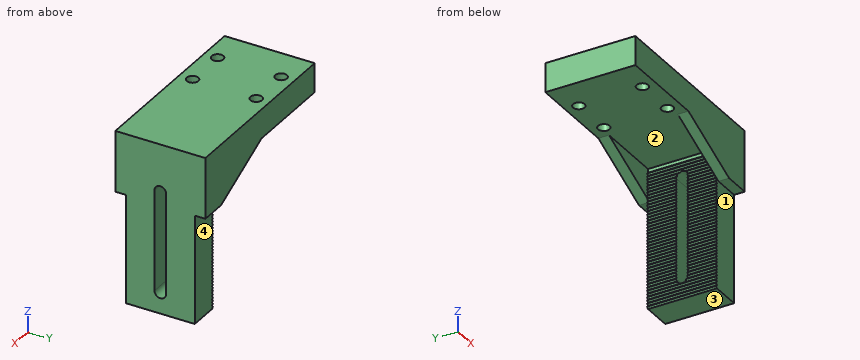
```python
from build123d import *

# Parameters (mm, degrees)
EXTRUDE_1_DEPTH          = 17
SKETCH_4_R               = 1.1
CUT_EXTRUDE_2_DEPTH      = 51.378566871
SKETCH_8_W               = 20.5
SKETCH_8_H               = 2
CUT_EXTRUDE_5_DEPTH      = 48.042533945
EXTRUDE_2_DEPTH          = 13
CUT_EXTRUDE_4_DEPTH      = 10
CUT_EXTRUDE_4_DEPTH_BACK = 48.042533945
EXTRUDE_3_DEPTH          = 2
EXTRUDE_4_DEPTH          = 2


with BuildPart() as part:
    # 草图1 → 凸台-拉伸1 (new body)
    with BuildSketch(Plane(origin=(0, 0, 0), x_dir=(1, 0, 0), z_dir=(0, 1, 0))):
        Polygon((0, 0), (-35, 0), (-35, 5.5), (-5, 5.5), (-5, 32), (0, 32), align=None)
    extrude(amount=EXTRUDE_1_DEPTH)

    # 草图4 → 切除-拉伸2 (cut, through all)
    with BuildSketch(Plane.XY):
        with Locations((-28.5, 14.5)):
            Circle(SKETCH_4_R)
        with Locations((-20.5, 14.5)):
            Circle(SKETCH_4_R)
        with Locations((-28.5, 2.5)):
            Circle(SKETCH_4_R)
        with Locations((-20.5, 2.5)):
            Circle(SKETCH_4_R)
    extrude(amount=-CUT_EXTRUDE_2_DEPTH, mode=Mode.SUBTRACT)

    # 草图8 → 切除-拉伸5 (cut, through all)
    with BuildSketch(Plane.ZY.offset(5)):
        with Locations((-21.75, 16)):
            Rectangle(SKETCH_8_W, SKETCH_8_H)
        with Locations((-21.75, 1)):
            Rectangle(SKETCH_8_W, SKETCH_8_H)
    extrude(amount=-CUT_EXTRUDE_5_DEPTH, mode=Mode.SUBTRACT)

    # 草图11 → 凸台-拉伸2 (add)
    with BuildSketch(Plane.XZ.offset(-2)):
        Polygon((-5, -5.5), (-5, -32), (-5.5, -32), (-5.8, -31.7), (-5.5, -31.4), (-5.8, -31.1), (-5.5, -30.8), (-5.8, -30.5), (-5.5, -30.2), (-5.8, -29.9), (-5.5, -29.6), (-5.8, -29.3), (-5.5, -29), (-5.8, -28.7), (-5.5, -28.4), (-5.8, -28.1), (-5.5, -27.8), (-5.8, -27.5), (-5.5, -27.2), (-5.8, -26.9), (-5.5, -26.6), (-5.8, -26.3), (-5.5, -26), (-5.8, -25.7), (-5.5, -25.4), (-5.8, -25.1), (-5.5, -24.8), (-5.8, -24.5), (-5.5, -24.2), (-5.8, -23.9), (-5.5, -23.6), (-5.8, -23.3), (-5.5, -23), (-5.8, -22.7), (-5.5, -22.4), (-5.8, -22.1), (-5.5, -21.8), (-5.8, -21.5), (-5.5, -21.2), (-5.8, -20.9), (-5.5, -20.6), (-5.8, -20.3), (-5.5, -20), (-5.8, -19.7), (-5.5, -19.4), (-5.8, -19.1), (-5.5, -18.8), (-5.8, -18.5), (-5.5, -18.2), (-5.8, -17.9), (-5.5, -17.6), (-5.8, -17.3), (-5.5, -17), (-5.8, -16.7), (-5.5, -16.4), (-5.8, -16.1), (-5.5, -15.8), (-5.8, -15.5), (-5.5, -15.2), (-5.8, -14.9), (-5.5, -14.6), (-5.8, -14.3), (-5.5, -14), (-5.8, -13.7), (-5.5, -13.4), (-5.8, -13.1), (-5.5, -12.8), (-5.8, -12.5), (-5.5, -12.2), (-5.8, -11.9), (-5.5, -11.6), (-5.8, -11.3), (-5.5, -11), (-5.8, -10.7), (-5.5, -10.4), (-5.8, -10.1), (-5.5, -9.8), (-5.8, -9.5), (-5.5, -9.2), (-5.8, -8.9), (-5.5, -8.6), (-5.8, -8.3), (-5.5, -8), (-5.8, -7.7), (-5.5, -7.4), (-5.8, -7.1), (-5.5, -6.8), (-5.8, -6.5), (-5.5, -6.2), (-5.5, -5.5), align=None)
    extrude(amount=-EXTRUDE_2_DEPTH)

    # 草图6 → 切除-拉伸4 (cut, two sides: drawn at the far end of the back side and taken through both)
    with BuildSketch(Plane.ZY.offset(5).offset(-CUT_EXTRUDE_4_DEPTH_BACK)):
        with BuildLine():
            Line((-28, 9.6), (-9, 9.6))
            ThreePointArc((-9, 9.6), (-7.9, 8.5), (-9, 7.4))
            Line((-9, 7.4), (-28, 7.4))
            ThreePointArc((-28, 7.4), (-29.1, 8.5), (-28, 9.6))
        make_face()
    extrude(amount=CUT_EXTRUDE_4_DEPTH + CUT_EXTRUDE_4_DEPTH_BACK, mode=Mode.SUBTRACT)

    # 草图12 → 凸台-拉伸3 (add)
    with BuildSketch(Plane.XZ):
        Polygon((-5, -11.5), (-5, -5.5), (-18, -5.5), align=None)
    extrude(amount=-EXTRUDE_3_DEPTH)

    # 草图13 → 凸台-拉伸4 (add)
    with BuildSketch(Plane(origin=(0, 17, 0), x_dir=(1, 0, 0), z_dir=(0, 1, 0))):
        Polygon((-5, 11.5), (-5, 5.5), (-18, 5.5), align=None)
    extrude(amount=-EXTRUDE_4_DEPTH)


solid = part.part
```
CAD build for the part. Positions are in the model's coordinates, mm. Face numbers are marked on the shaded views. Round coordinates to 2 decimals unless told otherwise and drop trailing zeros. Loops run counter-clockwise (first coordinate to the right, second up) from the corner with the lowest first, then second, coordinate; pieces in that order, holes last. Notation, with made-up numbers: M 54.5,48.25 L 76.5,48.25 A15 cw 76.5,69.25 Z; hole C -10.75,23 d2. An arc over 180 degrees is marked long. Use a Markdown table: item, result. Add a question column.
(1) Cut at D-D (y = 14). State how many separate pieces and enclosed holes the cut face has, and give its area (3 significant figures).
(2) Cut at B-B (z = -2). Give the cut face in (x, y), and give its area (3 significant figures).
(3) Pull direction Y, two halves, no side cores. Call the marked faces 1, 2, 3 and 4: +Y half, -Y half, draft (parallel to the pull), parting line (faces both ways), or undercut.
(4) Cut at C-C (x = -7.5). Give the cut face in (y, z).
(5) Flat gauge pins, fed straight in: pin 1 (4 mm diameter, centred on y = 9, z = -11.5, fed in from -X); pin 2 (1 mm diameter, centred on x = -24, y = 8.5, fed in from +Z); pin 3 (2.5 mm diameter, centred on x = -20.5, y = 14.5, fed in from -Z); pin 4 (2 mm diameter, centred on x = -28.5, y = 14.5, fed in from +Z). Where does each tip first touch, or does it go through?
(6) Cut at A-A (x = -20.5). Give the cut face in (y, z), and give its area (3 significant figures).
(7) Drill centre lines: line 1 (Y direction, x = -20.5, z = -3.4); line 2 (Y direction, x = -21.5, z = -3.5); line 3 (Y direction, x = -5.5, z = -18.5). Where is each one in solid material? Low to high.
Geometry says:
| question | item | result |
|---|---|---|
| 1 | separate pieces | 3 |
| 1 | enclosed holes | 0 |
| 1 | area | 321 mm² |
| 2 | outline | M -35,0 L 0,0 L 0,17 L -35,17 Z; hole C -28.5,2.5 d2.2; hole C -28.5,14.5 d2.2; hole C -20.5,2.5 d2.2; hole C -20.5,14.5 d2.2 |
| 2 | area | 580 mm² |
| 3 | face 1 | -Y half |
| 3 | face 2 | undercut |
| 3 | face 3 | draft |
| 3 | face 4 | +Y half |
| 4 | outline | M 0,-10.35 L 2,-10.35 L 2,-5.5 L 15,-5.5 L 15,-10.35 L 17,-10.35 L 17,0 L 0,0 Z |
| 5 | pin 1 | stops at x = -5.8 |
| 5 | pin 2 | stops at z = 0 |
| 5 | pin 3 | stops at z = -5.5 |
| 5 | pin 4 | passes through |
| 6 | outline | M 0,-5.5 L 1.4,-5.5 L 1.4,0 L 0,0 Z; M 3.6,-5.5 L 13.4,-5.5 L 13.4,0 L 3.6,0 Z; M 15.6,-5.5 L 17,-5.5 L 17,0 L 15.6,0 Z |
| 6 | area | 69.3 mm² |
| 7 | line 1 | y = 0 to 1.4, 3.6 to 13.4, 15.6 to 17 |
| 7 | line 2 | y = 0 to 2.04, 2.96 to 14.04, 14.96 to 17 |
| 7 | line 3 | y = 2 to 7.4, 9.6 to 15 |
